Build history of the part. All positions in model axes, mm. Give positions to 0.01 mm unless a question says otherwise; leave off trailing zeros. Write each loop counter-clockwise with the first axis right and the second up, starting at its lowest first coordinate (ties: lowest second). Pieces come first, ordered by that corner, then holes. Notation, with made-up numbers: M 0.25,-0.75 L 22.25,-0.75 A3 ccw 22.25,4.25 Z; hole C -21,-12 d9. An arc over 180 degrees is marked long. Return JSON: item names as keys, results as strings. Group by question number.
Q1. Band-saw the part on C-C, the plane z = -9.5. Give the cut face in (x, y), then the cut area to 3 significant figures.
Q2. Wall check: probe 1 along Y at (x, z) = (114.5, 1.5); probe 2 along Y at (x, z) = (26.5, -5); probe 3 along Y at (x, z) = (55, -15). Give the ranges that are in metal, low to high.
Q3. Flat gauge pins, fed straight in: pin 1 Ø1 at (x, z) = (22, -2.5) entering from -Y; pin 2 Ø4 at (x, z) = (108, 3.5) entering from -Y; pin 3 Ø6 at (x, z) = (114.5, -2) entering from -Y; pin 4 Ø7.5 at (y, z) = (7.57, 0) entering from +X. Where does each tip first touch, or does it go through?
Q4. Band-saw the part on B-B, the plane y = -73.5. Give the cut face in (x, z).
Q5. Band-saw the part on A-A, the plane x = 73. Give the cut face in (y, z), then the cut area to 3 significant figures.
Q6. Pull direction Y, two halves, no side cores. Call faces 1 (the flat face through (69, 45.672, -1)), 2 (the cylindrical face through (68.87, -37.36, -2.43)), 3 (the flat face through (68.872, -97.516, 6.386)): +Y half, -Y half, draft (parallel to the pull), parting line (faces both ways), or undercut.
from build123d import *

# Parameters (mm, degrees)
F0_R     = 6.35
F1_DEPTH = 139.7


with BuildPart() as f1:
    # F0 (on Right) → F1 (new body)
    with BuildSketch(Plane.YZ):
        Polygon((45.672475, -17.78), (45.672475, 16.51), (-111.807525, 16.51), (-101.070702, 12.595123), (-111.807525, 12.595123), (-82.819068, 0), (-62.477541, -17.78), align=None)
        with Locations((-43.227525, 0)):
            Circle(F0_R, mode=Mode.SUBTRACT)
        with Locations((7.572475, 0)):
            Circle(F0_R, mode=Mode.SUBTRACT)
    extrude(amount=F1_DEPTH)


solid = f1.part
From the geometry:
{
 "1": {"outline": "M 0,-71.95 L 139.7,-71.95 L 139.7,45.67 L 0,45.67 Z", "area": "16,400 mm^2"},
 "2": {"probe 1": "y = -86.27 to -49.4, -37.06 to 1.4, 13.74 to 45.67", "probe 2": "y = -77.1 to -47.14, -39.31 to 3.66, 11.49 to 45.67", "probe 3": "y = -65.66 to 45.67"},
 "3": {"pin 1": "stops at y = -80.53", "pin 2": "stops at y = -95.48", "pin 3": "stops at y = -85.12", "pin 4": "passes through"},
 "4": {"outline": "M 0,-8.15 L 139.7,-8.15 L 139.7,16.51 L 0,16.51 Z"},
 "5": {"outline": "M -111.81,12.6 L -82.82,0 L -62.48,-17.78 L 45.67,-17.78 L 45.67,16.51 L -111.81,16.51 L -101.07,12.6 Z; hole C -43.23,0 d12.7; hole C 7.57,0 d12.7", "area": "4,250 mm^2"},
 "6": {"face 1": "+Y half", "face 2": "undercut", "face 3": "-Y half"}
}
